from build123d import *

# Parameters (mm, degrees)
BOSS_EXTRUDE1_DEPTH = 5.08
SKETCH9_W           = 4.318
SKETCH9_H           = 4.318
CUT_EXTRUDE3_DEPTH  = 1.778
SKETCH10_W          = 4.318
SKETCH10_H          = 4.318
CUT_EXTRUDE4_DEPTH  = 1.778
SKETCH11_W          = 4.318
SKETCH11_H          = 4.318
CUT_EXTRUDE5_DEPTH  = 1.778
SKETCH12_W          = 4.318
SKETCH12_H          = 4.318
CUT_EXTRUDE6_DEPTH  = 1.778


with BuildPart() as part:
    # Sketch1 → Boss-Extrude1 (new body)
    with BuildSketch(Plane(origin=(0, 0, 0), x_dir=(1, 0, 0), z_dir=(0, 1, 0))):
        Polygon((-28.91784315, -24.413806508), (-16.791726333, 63.108386813), (-104.313919654, 75.23450363), (-116.440036471, -12.287689691), align=None)
        Polygon((-20.806654289, 60.039384261), (-101.244917102, 71.219575674), (-112.425108515, -9.218687139), (-31.986845702, -20.398878552), align=None, mode=Mode.SUBTRACT)
    extrude(amount=BOSS_EXTRUDE1_DEPTH)

    # Sketch9 → Cut-Extrude3 (cut)
    with BuildSketch(Plane(origin=(-3.387750967, 0, 24.3738942), x_dir=(-0.9904784923139263, 0, -0.13766755704788136), z_dir=(0.13766755704788133, 0, -0.9904784923139262))):
        with Locations((43.18, 3.81)):
            Rectangle(SKETCH9_W, SKETCH9_H)
    extrude(amount=-CUT_EXTRUDE3_DEPTH, mode=Mode.SUBTRACT)

    # Sketch10 → Cut-Extrude4 (cut)
    with BuildSketch(Plane(origin=(7.792440446, 0, -56.064368613), x_dir=(0.9904784923139262, 0, 0.1376675570478817), z_dir=(-0.1376675570478817, 0, 0.9904784923139263))):
        with Locations((-43.18, 3.81)):
            Rectangle(SKETCH10_W, SKETCH10_H)
    extrude(amount=-CUT_EXTRUDE4_DEPTH, mode=Mode.SUBTRACT)

    # Sketch11 → Cut-Extrude5 (cut)
    with BuildSketch(Plane(origin=(7.792440446, 0, -56.064368613), x_dir=(0.9904784923139262, 0, 0.1376675570478817), z_dir=(-0.1376675570478817, 0, 0.9904784923139263))):
        with Locations((-95.758, 3.81)):
            Rectangle(SKETCH11_W, SKETCH11_H)
    extrude(amount=-CUT_EXTRUDE5_DEPTH, mode=Mode.SUBTRACT)

    # Sketch12 → Cut-Extrude6 (cut)
    with BuildSketch(Plane(origin=(-3.387750967, 0, 24.3738942), x_dir=(-0.9904784923139263, 0, -0.13766755704788136), z_dir=(0.13766755704788133, 0, -0.9904784923139262))):
        with Locations((95.758, 3.81)):
            Rectangle(SKETCH12_W, SKETCH12_H)
    extrude(amount=-CUT_EXTRUDE6_DEPTH, mode=Mode.SUBTRACT)


solid = part.part
The listing builds one solid part. Answer for the finished solid, in the listing's coordinates (mm). A direction names the side the tool comes from. Give positions to 0.01 mm unless a question says otherwise; leave off trailing zeros. Write each loop counter-clockwise with the first axis right and the second up, starting at its lowest first coordinate (ties: lowest second). Pieces come first, ordered by that corner, then holes.
Item 1: Determine the mould class of faces 1 (the flat face through (-63.2, 0, -66.2)), 2 (the flat face through (-46.371, 3.39, 20.195)), 3 (the flat face through (-35, 1.651, -63)), 4 (the flat face through (-73.292, 2.504, 18.266)) for opening direction Z: released by +Z, released by -Z, zero draft, split by the parting line, or undercut.
Item 2: Section C-C, the plane z = -36 is taken. Write down the section's boundary in (x, y).
Item 3: Section B-B, the plane x = -24 is taken. Write down the section's boundary in (y, z), plus the area to 3 significant figures.
Item 4: Find the intervals of material crossed by line 1 along Z through (x, y) = (-86, 1.7); line 2 along Z through (x, y) = (-49, 3.5); line 3 along X through (y, z) = (4.2, -13.5), in increasing order.
Item 5: Flat-ended cylindrical pins translate along their axes: P1, Ø2, axis at y = 1.5, z = -63.5, coming from the -X side; P2, Ø1.9, axis at x = -98, z = 11.5, coming from the +Y side; P3, Ø1, axis at y = 2.5, z = -3.5, coming from the +X side. Find the tip coordinate at first contact, or state that the pin passes through.
Item 6: Section A-A, the plane y = 4 is taken. Write down the section's boundary in (x, z), plus the area to 3 significant figures.
Item 7: Section D-D, the plane x = -46 is taken. Write down the section's boundary in (y, z), plus the area to 3 significant figures.
Item 8: Which of the six approach directions +Z, -Z, +X, -X, +Y, -Y give full straight-line access (tool end or side, diameter ignored) to faces 5 (the flat face through (-60.46, 2.5, -65.55)), 6 (the flat face through (-86.839, 3.39, -71.012)), 7 (the flat face through (-59.94, 2.504, -69.087))?
Completed:
1. face 1: zero draft
1. face 2: undercut
1. face 3: undercut
1. face 4: released by +Z
2. outline: (-109.75, 0) - (-106.14, 0) - (-106.14, 5.08) - (-109.75, 5.08) - close; (-24.15, 0) - (-20.55, 0) - (-20.55, 5.08) - (-24.15, 5.08) - close
3. outline: (0, -64.11) - (5.08, -64.11) - (5.08, -60.48) - (0, -60.48) - close; (0, -37.06) - (5.08, -37.06) - (5.08, -11.08) - (0, -11.08) - close
3. area: 150 mm2
4. line 1: z = -72.7 to -70.9, 12.89 to 16.51
4. line 2: z = -67.57 to -63.96, 18.03 to 21.63
4. line 3: x = -112.87 to -109.27, -27.28 to -23.66
5. P1: stops at x = -106.08
5. P2: stops at y = 1.65
5. P3: stops at x = -24.98
6. outline: (-116.44, 12.29) - (-104.31, -75.23) - (-16.79, -63.11) - (-28.92, 24.41) - close; hole (-112.43, 9.22) - (-101.24, -71.22) - (-89.19, -69.54) - (-88.95, -71.31) - (-84.67, -70.71) - (-84.92, -68.95) - (-37.11, -62.31) - (-36.87, -64.07) - (-32.59, -63.47) - (-32.84, -61.71) - (-20.81, -60.04) - (-31.99, 20.4) - (-44.02, 18.73) - (-44.26, 20.49) - (-48.54, 19.89) - (-48.3, 18.13) - (-96.1, 11.49) - (-96.34, 13.25) - (-100.62, 12.65) - (-100.37, 10.89) - close
6. area: 1,180 mm2
7. outline: (0, -67.16) - (5.08, -67.16) - (5.08, -63.54) - (0, -63.54) - close; (0, 18.45) - (1.65, 18.45) - (1.65, 20.25) - (5.08, 20.25) - (5.08, 22.05) - (0, 22.05) - close
7. area: 30.5 mm2
8. face 5: +Y, -Y
8. face 6: +Y
8. face 7: -Z, +X, +Y, -Y
